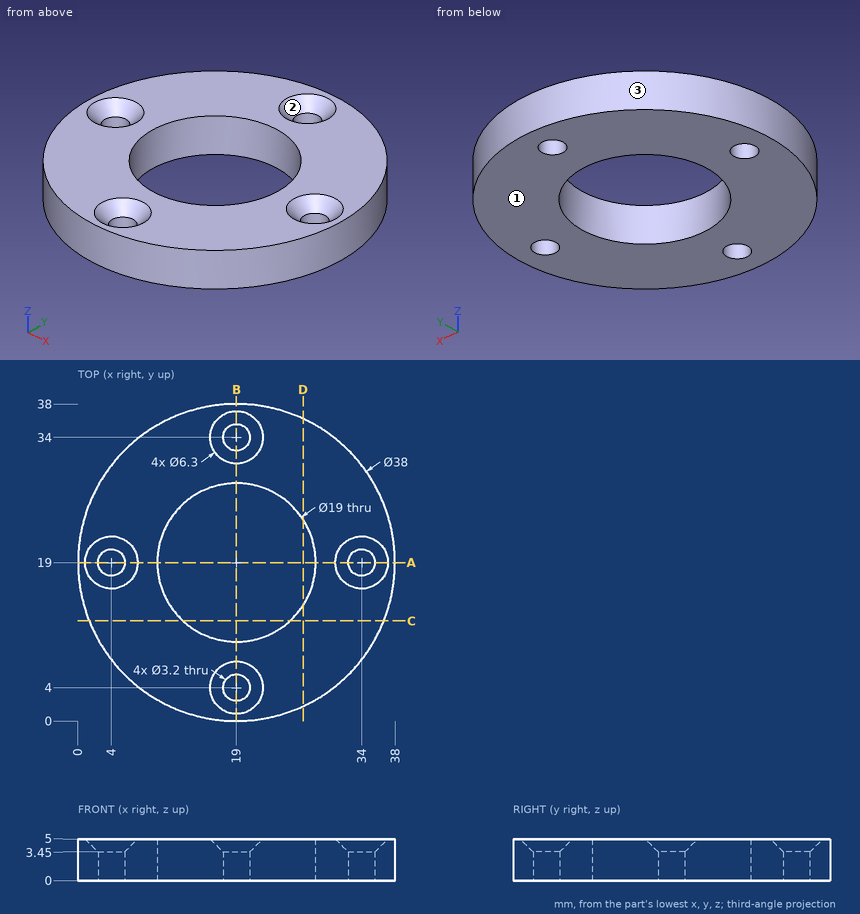
Design review of the part shown in the three views and the two pictorial views. Dimensions are in mm from the part's minimum x, y and z. Give positions to 0.01 mm unless a question says otherwise; leave off trailing zeros. Loops run counter-clockwise (first coordinate to the right, second up) from the corner with the lowest first, then second, coordinate; pieces in that order, holes last. Notation, with made-up numbers: M -30,-39.75 L -7,-39.75 A24 cw -7,-3.75 Z; hole C -9.75,37 d4. An arc over 180 degrees is marked long. Put each result on its own line as item: value. Start each with the question number.
(1) Add section D-D, the plane x = 27. Write out the cut boundary in (y, z).
(2) Wall thickness on L1, parallel to Y at x = 19, z = 1.1; L2, parallel to Y at x = 22, z = 1.05; L3, parallel to Y at x = 34, z = 4: over which ranges is each line inside the solid? List them lowest first.
(3) For pin 1 (5 mm diameter, centred on x = 19, y = 4, fed in from +Z); pin 2 (2 mm diameter, centred on x = 6, z = 3.5, fed in from -Y); pin 3 (1.5 mm diameter, centred on y = 26, z = 4, fed in from +X), all flat-tipped, find the tip position at first contact; note any pin that passes through.
(4) Add section C-C, the plane y = 12. Write out the cut boundary in (x, z), then the cut area to 3 significant figures.
(5) The part is to be moulded in two halves that separate along Y. For the marked faces 1, 2 and 3, say which applies: +Y half, -Y half, draft (parallel to the pull), parting line (faces both ways), or undercut.
(6) Add section A-A, the plane y = 19. Write out the cut boundary in (x, z), then the cut area to 3 significant figures.
Result:
1. outline: M 1.77,0 L 13.88,0 L 13.88,5 L 1.77,5 Z; M 24.12,0 L 36.23,0 L 36.23,5 L 24.12,5 Z
2. L1: y = 0 to 2.4, 5.6 to 9.5, 28.5 to 32.4, 35.6 to 38
2. L2: y = 0.24 to 9.99, 28.01 to 37.76
2. L3: y = 7.34 to 16.85, 21.15 to 30.66
3. pin 1: stops at z = 4.35
3. pin 2: stops at y = 4.27
3. pin 3: stops at x = 36.94
4. outline: M 1.34,0 L 12.58,0 L 12.58,5 L 1.34,5 Z; M 25.42,0 L 36.66,0 L 36.66,5 L 25.42,5 Z
4. area: 112 mm^2
5. face 1: draft
5. face 2: undercut
5. face 3: parting line
6. outline: M 0,0 L 2.4,0 L 2.4,3.45 L 0.85,5 L 0,5 Z; M 5.6,0 L 9.5,0 L 9.5,5 L 7.15,5 L 5.6,3.45 Z; M 28.5,0 L 32.4,0 L 32.4,3.45 L 30.85,5 L 28.5,5 Z; M 35.6,0 L 38,0 L 38,5 L 37.15,5 L 35.6,3.45 Z
6. area: 58.2 mm^2
